For this review, take the finished solid that the model builds, in its own axes (mm). Round coordinates to 2 decimals unless told otherwise and drop trailing zeros. Order: outer loops, then holes, each group sorted by start corner. A loop starts at its lowest first (then second) coordinate and runs counter-clockwise, first axis right, second up. Notation, with made-up numbers: M -18.5,-18.5 L -14.5,-18.5 A18 ccw -14.5,-13.5 Z; hole C 14,61.5 d1. An arc over 180 degrees is marked long. Put each result on its own line as item: value.
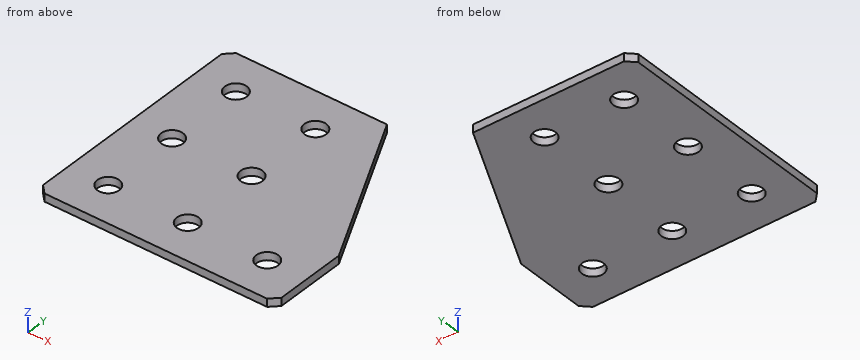
from build123d import *

# Parameters (mm, degrees)
EXTRUDE_1_DEPTH   = 2
HOLE_WIZARD_M51_D = 5.5
CHAMFER_1_SIZE    = 2


with BuildPart() as part:
    # Эскиз1 → Бобышка-Вытянуть1 (new body)
    with BuildSketch(Plane(origin=(0, 0, 0), x_dir=(1, 0, 0), z_dir=(0, 0, -1))):
        Polygon((0, 0), (0, 60), (60, 60), (60, 40), (40, 0), align=None)
    extrude(amount=EXTRUDE_1_DEPTH)

    # Отверстие с зазором M51 (through all)
    with Locations(Plane(origin=(0, 0, -2), x_dir=(1, 0, 0), z_dir=(0, 0, -1))):
        with Locations((30, 50), (10, 50), (10, 30), (10, 10), (50, 50), (30, 30), (30, 10)):
            Hole(HOLE_WIZARD_M51_D / 2)

    # Фаска1
    chamfer_1_edges = [part.edges().sort_by_distance(p)[0] for p in [
        (0, 0, -1),
        (0, -60, -1),
        (60, -60, -1),
    ]]
    chamfer(chamfer_1_edges, length=CHAMFER_1_SIZE)


solid = part.part
(1) Add section A-A on y = -30. Give the boundary of the cut face in (x, z).
A:
outline: M 0,-2 L 7.25,-2 L 7.25,0 L 0,0 Z; M 12.75,-2 L 27.25,-2 L 27.25,0 L 12.75,0 Z; M 32.75,-2 L 55,-2 L 55,0 L 32.75,0 Z
(2) Add section D-D on y = -50. Give the boundary of the cut face in (x, z).
A:
outline: M 0,-2 L 7.25,-2 L 7.25,0 L 0,0 Z; M 12.75,-2 L 27.25,-2 L 27.25,0 L 12.75,0 Z; M 32.75,-2 L 47.25,-2 L 47.25,0 L 32.75,0 Z; M 52.75,-2 L 60,-2 L 60,0 L 52.75,0 Z
(3) To check wall thickness, follow L1, parallel to Y at x = 10, z = -0.8; L2, parallel to X at y = -50, z = -0.8; L3, parallel to Y at x = 32, z = -1.55. State the ranges of each line that lie inside material, in increasing order.
A:
L1: y = -60 to -52.75, -47.25 to -32.75, -27.25 to -12.75, -7.25 to 0
L2: x = 0 to 7.25, 12.75 to 27.25, 32.75 to 47.25, 52.75 to 60
L3: y = -60 to -51.89, -48.11 to -31.89, -28.11 to -11.89, -8.11 to 0
(4) Add section C-C on z = -0.55. Give the boundary of the cut face in (x, y), then the cut area to 3 significant figures.
A:
outline: M 0,-58 L 2,-60 L 58,-60 L 60,-58 L 60,-40 L 40,0 L 2,0 L 0,-2 Z; hole C 10,-50 d5.5; hole C 10,-30 d5.5; hole C 10,-10 d5.5; hole C 30,-50 d5.5; hole C 30,-30 d5.5; hole C 30,-10 d5.5; hole C 50,-50 d5.5
area: 3,030 mm2
(5) Add section B-B on x = 10. Give the boundary of the cut face in (y, z).
A:
outline: M -60,-2 L -52.75,-2 L -52.75,0 L -60,0 Z; M -47.25,-2 L -32.75,-2 L -32.75,0 L -47.25,0 Z; M -27.25,-2 L -12.75,-2 L -12.75,0 L -27.25,0 Z; M -7.25,-2 L 0,-2 L 0,0 L -7.25,0 Z
